Autodesk Inventor part; units mm, degrees
ref_plane "YZ Plane" through (0, 0, 0) normal (1, 0, 0) x (0, 1, 0)
ref_plane "XZ Plane" through (0, 0, 0) normal (0, 1, 0) x (-1, 0, 0)
ref_plane "XY Plane" through (0, 0, 0) normal (0, 0, 1) x (1, 0, 0)
sketch "Sketch1" plane through (0, 0, 0) normal (0, 0, 1) x (1, 0, 0)
  circle A0 centre (0, 0) radius 18
  dimension "d0" = 36
extrude "Extrusion1" add sketch "Sketch1" along normal blind 2.5
sketch "Sketch2" plane through (0, 0, 2.5) normal (0, 0, 1) x (1, 0, 0)
  line L0 (0, 0) -> (0, 11)
  circle A0 centre (0, 11) radius 1.25
  circle A1 centre (0, 0) radius 5
  circle A2 centre (7.7782, 7.7782) radius 1.25
  circle A3 centre (11, 0) radius 1.25
  circle A4 centre (7.7782, -7.7782) radius 1.25
  circle A5 centre (0, -11) radius 1.25
  circle A6 centre (-7.7782, -7.7782) radius 1.25
  circle A7 centre (-11, 0) radius 1.25
  circle A8 centre (-7.7782, 7.7782) radius 1.25
  dimension "d3" = 11
  dimension "d4" = 2.5
  dimension "d5" = 10
  dimension "d8" = 360
extrude "Extrusion2" cut sketch "Sketch2" against normal through all
sketch "Sketch3" plane through (0, 0, 2.5) normal (0, 0, 1) x (1, 0, 0)
  circle A0 centre (0, 0) radius 15
  circle A1 centre (0, 0) radius 18
  dimension "d12" = 30
extrude "Extrusion3" cut sketch "Sketch3" against normal through all
sketch "Sketch4" plane through (0, 0, 2.5) normal (0, 0, 1) x (1, 0, 0)
  circle A0 centre (0, 11) radius 1.25
  arc A1 (-2.1651, 9.75) -> (2.1651, 9.75) centre (0, 11) ccw
  circle A2 centre (-7.7782, 7.7782) radius 1.25
  circle A3 centre (7.7782, 7.7782) radius 1.25
  circle A4 centre (0, 0) radius 5
  line L0 (2.1651, 9.75) -> (6.1129, 13.6979)
  circle A5 centre (0, 0) radius 15
  line L1 (2.1651, 9.75) -> (7.7482, 9.75) construction
  line L2 (-2.1651, 9.75) -> (-6.1129, 13.6979)
  line L3 (-2.1651, 9.75) -> (3.4181, 9.75) construction
  arc A6 (6.1129, 13.6979) -> (-6.1129, 13.6979) centre (0, 0) ccw
  dimension "d15" = 5
  dimension "d17" = 45
  dimension "d18" = 135
extrude "Extrusion4" cut sketch "Sketch4" against normal blind 10 contours L2 A5 L0 A1 picked at (3.4839, 13.2226)
fillet "Fillet1" radius 2 4 edges at (-6.1129, 13.6979, 1.25) (6.1129, 13.6979, 1.25) (-2.1651, 9.75, 1.25) (2.1651, 9.75, 1.25)
sketch "Sketch5" plane through (0, 0, 2.5) normal (0, 0, 1) x (1, 0, 0)
  line L0 (0, 0) -> (1, 0)
  line L1 (1, 0) -> (1, 1)
  line L2 (1, 1) -> (0, 1)
  line L3 (0, 1) -> (0, 0)
  dimension "d22" = 1
  dimension "d23" = 1
extrude "Extrusion5" add sketch "Sketch5" along normal blind 1
sketch "Sketch6" plane through (0, 1, 2.5) normal (0, 1, 0) x (1, 0, 0)
  line L0 (2.0766, 0) -> (-2.0766, 0)
  line L1 (-15, 2.5) -> (-15, 0)
  line L2 (0, 0) -> (-15, 0)
  line L3 (-15, 0) -> (-15, 0.5)
  line L4 (-15, 0.5) -> (0, 0.5)
  line L5 (0, 0.5) -> (0, 0)
  line L6 (0, 0) -> (15, 0)
  line L7 (15, 0) -> (15, 0.5)
  line L8 (15, 0.5) -> (0, 0.5)
  line L9 (0, 0.5) -> (0, 0)
  point P0 (0, 2.5)
  point P1 (0, 0.5)
  dimension "d26" = 0.5
  dimension "d27" = 15
extrude "Extrusion6" cut sketch "Sketch6" along normal through all both and the other way through all
sketch "Sketch7" plane through (0, 0, 3.5) normal (0, 0, 1) x (1, 0, 0)
  line L0 (1, 1) -> (0, 1)
  line L1 (0, 0) -> (1, 0)
  line L2 (0, 1) -> (1, 1)
  line L3 (1, 1) -> (1, 0)
  line L4 (1, 0) -> (0, 0)
  line L5 (0, 0) -> (0, 1)
extrude "Extrusion7" cut sketch "Sketch7" against normal blind 1
sketch "Sketch8" plane through (0, 0, 2) normal (0, 0, 1) x (1, 0, 0)
  circle A0 centre (0, 0) radius 5.25
  dimension "d32" = 10.5
extrude "Extrusion8" cut sketch "Sketch8" against normal through all
sketch "Sketch9" plane through (0, 0, 0) normal (0, 0, -1) x (-1, 0, 0)
  circle A0 centre (0, -11) radius 1.25
  circle A1 centre (0, -11) radius 1.35
  circle A2 centre (-7.7782, -7.7782) radius 1.25
  circle A3 centre (-7.7782, -7.7782) radius 1.35
  circle A4 centre (-11, 0) radius 1.25
  circle A5 centre (-11, 0) radius 1.35
  circle A6 centre (-7.7782, 7.7782) radius 1.25
  circle A7 centre (-7.7782, 7.7782) radius 1.35
  circle A8 centre (7.7782, -7.7782) radius 1.25
  circle A9 centre (7.7782, -7.7782) radius 1.35
  circle A10 centre (11, 0) radius 1.25
  circle A11 centre (11, 0) radius 1.35
  circle A12 centre (7.7782, 7.7782) radius 1.25
  circle A13 centre (7.7782, 7.7782) radius 1.35
  point P0 (0, 0)
  dimension "d35" = 2.7
  dimension "d36" = 2.7
  dimension "d37" = 2.7
  dimension "d38" = 2.7
  dimension "d39" = 2.7
  dimension "d40" = 2.7
  dimension "d41" = 2.7
extrude "Extrusion9" cut sketch "Sketch9" against normal through all contours A1 | A3 | A5 | A7 | A9 | A10 | A11
properties part number "Pulley_middle"
Design review of the part built by this model. Coordinates are the model's own, in mm. A direction names the side the tool comes from. Coordinates: 2 decimals unless noted, no trailing zeros. Order: outer loops, then holes, each group sorted by start corner. A loop starts at its lowest first (then second) coordinate and runs counter-clockwise, first axis right, second up.
1) Mouldability with a two-part tool opening along Y and no side actions: class faces 1 (the cylindrical face through (8.773, -6.866, 0.986)), 2 (the cylindrical face through (-6.624, 7.299, 1.014)), 3 (the flat face through (4, -4, 2)), 4 (the cylindrical face through (0, 8.5, 1)) as +Y half, -Y half, draft (parallel to the pull), parting line (faces both ways), or undercut.
2) Take a section at D-D, the plane z = 1.35. State how many separate pieces and enclosed holes the cut face has, and give its area (3 significant figures).
3) Take a section at B-B, the plane y = 0. Give the boundary of the cut face in (x, z).
4) Clearance check with flat-ended pins moving along their axes: pin 1 (2 mm diameter, centred on x = 7.78, y = -7.78, fed in from -Z); pin 2 (3 mm diameter, centred on x = 0, y = -11, fed in from -Z). State where each tip first meets the part, or that it passes through.
5) For faces 5 (the flat face through (3.686, 11.271, 1.014)), 6 (the cylindrical face through (9.753, -0.517, 0.986)), list the 3-axis set-ups (+Z, -Z, +X, -X, +Y, -Y) from which the entire face can be reached by the end or side of a thin tool; tool diameter is ignored.
6) Take a section at A-A, the plane x = 0. Give the boundary of the cut face in (y, z), and give its area (3 significant figures).
7) Take a section at C-C, the plane x = 11. Give the boundary of the cut face in (y, z).
8) Wall thickness on line 1 along X through (y, z) = (-1, 1.65); line 2 along X through (y, z) = (-9, 1.15); line 3 along Y through (x, z) = (8.75, 1.45): over which ranges is each line inside the solid? List them lowest first.
Returned:
1. face 1: undercut
1. face 2: undercut
1. face 3: draft
1. face 4: +Y half
2. separate pieces: 1
2. enclosed holes: 8
2. area: 533 mm2
3. outline: (-15, 0) - (-12.35, 0) - (-12.35, 2) - (-15, 2) - close; (-9.65, 0) - (-5.25, 0) - (-5.25, 2) - (-9.65, 2) - close; (5.25, 0) - (9.65, 0) - (9.65, 2) - (5.25, 2) - close; (12.35, 0) - (15, 0) - (15, 2) - (12.35, 2) - close
4. pin 1: passes through
4. pin 2: stops at z = 0
5. face 5: +Z, -Z, +Y
5. face 6: +Z, -Z
6. outline: (-15, 0) - (-12.35, 0) - (-12.35, 2) - (-15, 2) - close; (-9.65, 0) - (-5.25, 0) - (-5.25, 2) - (-9.65, 2) - close; (5.25, 0) - (8.5, 0) - (8.5, 2) - (5.25, 2) - close
6. area: 20.6 mm2
7. outline: (-10.2, 0) - (-1.35, 0) - (-1.35, 2) - (-10.2, 2) - close; (1.35, 0) - (10.2, 0) - (10.2, 2) - (1.35, 2) - close
8. line 1: x = -14.97 to -11.91, -10.09 to -5.15, 5.15 to 10.09, 11.91 to 14.97
8. line 2: x = -12 to -8.35, -7.2 to 7.2, 8.35 to 12
8. line 3: y = -12.18 to -8.72, -6.84 to 6.84, 8.72 to 12.18
